Can you work these out from the model? Positions are in its coordinate system, mm. Face numbers are marked on the shaded views. Coordinates: 2 decimals unless noted, no trailing zeros. Order: outer loops, then holes, each group sorted by start corner. A loop starts at its lowest first (then second) coordinate and runs counter-clockwise, first axis right, second up. Notation, with made-up numbers: (9, 36) -> (35, 36) arc R31 cw to (35, 62) -> close; hole circle Ø5 at (-1, -36). An arc over 180 degrees is marked (long way). Answer in a Markdown table with one row per item. Add a question column.
1. We'd pull the mould along X, two halves only. Please class the marked faces 1, 2 and 3: pulls with the +X half, pulls with the -X half, needs draft (parallel to the pull), parting line crosses it, or undercut.
2. Imagine slicing it at A-A on x = 27. Write out the boundary of the cut face in (y, z), plus the area to 3 significant figures.
3. Will these pins go through, and if not, where does the flat tip stop? pin 1 (10 mm diameter, centred on x = 35.5, z = 80.5, fed in from +Y); pin 2 (4 mm diameter, centred on y = 13.5, z = 45, fed in from +X); pin 3 (2 mm diameter, centred on y = 64.5, z = 62.5, fed in from +X).
4. If I drill on line 1 along Y through (x, z) = (20, 29); line 2 along X through (y, z) = (26, 48); line 3 along Y through (x, z) = (42.5, 44), over which ranges is the centre line in solid material (lowest first)? Write a range as [from, to].
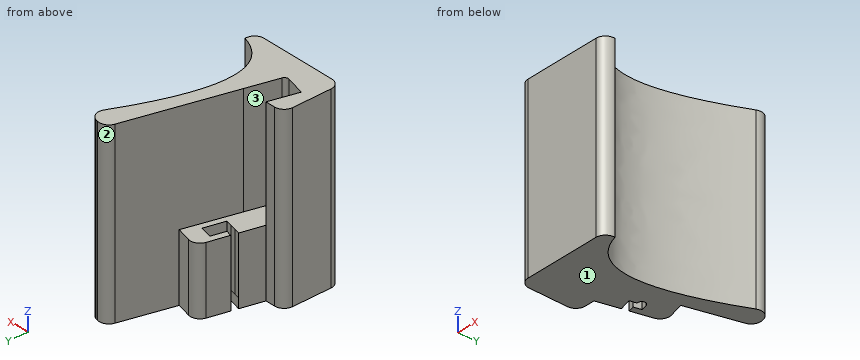
from build123d import *

# Parameters (mm, degrees)
BOSS_EXTRUDE1_DEPTH = 92
BOSS_EXTRUDE2_DEPTH = 5
BOSS_EXTRUDE3_START = 5
BOSS_EXTRUDE3_DEPTH = 30


with BuildPart() as part:
    # Sketch1 → Boss-Extrude1 (new body)
    with BuildSketch(Plane.XY):
        with BuildLine():
            Line((37.386921991, 84.40496063), (22.933554815, 30))
            Line((22.933554815, 30), (18.60433255, 13.818460639))
            ThreePointArc((18.60433255, 13.818460639), (17.672613775, 12.603502297), (16.154645697, 12.403510891))
            Line((16.154645697, 12.403510891), (6.013160809, 15.120913577))
            Line((6.013160809, 15.120913577), (10, 30))
            Line((10, 30), (5, 30))
            ThreePointArc((5, 30), (1.464466094, 28.535533906), (0, 25))
            Line((0, 25), (0, 5))
            ThreePointArc((0, 5), (1.464466094, 1.464466094), (5, 0))
            Line((5, 0), (44.402158914, 0))
            ThreePointArc((44.402158914, 0), (48.110924034, 1.646634335), (49.376897159, 5.501975487))
            add(Edge.make_bspline(
                [(47.769018508, 80.690333507), (37.23731495, 58.823324345), (26.973591169, 24.424922179), (38.309234052, 8.697752331), (49.376897159, 5.501975487)],
                knots=[0.034365073, 0.034365073, 0.034365073, 0.034365073, 0.450207032, 0.866048991, 0.866048991, 0.866048991, 0.866048991], degree=3))
            ThreePointArc((47.769018508, 80.690333507), (47.791234842, 84.982795953), (44.476941442, 87.710649813))
            Line((44.476941442, 87.710649813), (43.43198058, 87.971890028))
            ThreePointArc((43.43198058, 87.971890028), (39.678375933, 87.427416305), (37.386921991, 84.40496063))
        make_face()
    extrude(amount=BOSS_EXTRUDE1_DEPTH)

    # Sketch1_3 → Boss-Extrude2 (add)
    with BuildSketch(Plane.XY):
        with BuildLine():
            Line((22.933554815, 30), (30.160238403, 57.202480315))
            Line((30.160238403, 57.202480315), (22.508418768, 59.201215835))
            ThreePointArc((22.508418768, 59.201215835), (18.694880172, 58.664472736), (16.394052668, 55.576210673))
            Line((16.394052668, 55.576210673), (13.75675976, 45.027039041))
            Line((13.75675976, 45.027039041), (16.890316486, 44.243649859))
            Line((16.890316486, 44.243649859), (17.860458987, 48.12421986))
            Line((17.860458987, 48.12421986), (21.013422112, 47.335979078))
            ThreePointArc((21.013422112, 47.335979078), (22.468635862, 44.910622828), (20.043279612, 43.455409078))
            Line((20.043279612, 43.455409078), (19.194404924, 40.059910327))
            Line((19.194404924, 40.059910327), (12.907885073, 41.63154029))
            Line((12.907885073, 41.63154029), (10, 30))
            Line((10, 30), (6.013160809, 15.120913577))
            Line((6.013160809, 15.120913577), (16.154645697, 12.403510891))
            ThreePointArc((16.154645697, 12.403510891), (17.672613775, 12.603502297), (18.60433255, 13.818460639))
            Line((18.60433255, 13.818460639), (22.933554815, 30))
        make_face()
    extrude(amount=BOSS_EXTRUDE2_DEPTH)

    # Sketch1_4 → Boss-Extrude3 (add)
    with BuildSketch(Plane.XY.offset(BOSS_EXTRUDE3_START)):
        with BuildLine():
            Line((22.933554815, 30), (30.160238403, 57.202480315))
            Line((30.160238403, 57.202480315), (22.508418768, 59.201215835))
            ThreePointArc((22.508418768, 59.201215835), (18.694880172, 58.664472736), (16.394052668, 55.576210673))
            Line((16.394052668, 55.576210673), (14.72690226, 48.907609041))
            Line((14.72690226, 48.907609041), (13.75675976, 45.027039041))
            Line((13.75675976, 45.027039041), (16.890316486, 44.243649859))
            Line((16.890316486, 44.243649859), (17.860458987, 48.12421986))
            Line((17.860458987, 48.12421986), (18.709333674, 51.51971861))
            Line((18.709333674, 51.51971861), (25.015259925, 49.943237047))
            Line((25.015259925, 49.943237047), (22.34736805, 39.271669546))
            Line((22.34736805, 39.271669546), (19.194404924, 40.059910327))
            Line((19.194404924, 40.059910327), (16.041441799, 40.848151108))
            Line((16.041441799, 40.848151108), (12.907885073, 41.63154029))
            Line((12.907885073, 41.63154029), (10, 30))
            Line((10, 30), (6.013160809, 15.120913577))
            Line((6.013160809, 15.120913577), (16.154645697, 12.403510891))
            ThreePointArc((16.154645697, 12.403510891), (17.672613775, 12.603502297), (18.60433255, 13.818460639))
            Line((18.60433255, 13.818460639), (22.933554815, 30))
        make_face()
    extrude(amount=BOSS_EXTRUDE3_DEPTH)


solid = part.part
Answers follow:
| question | item | result |
|---|---|---|
| 1 | face 1 | needs draft |
| 1 | face 2 | parting line crosses it |
| 1 | face 3 | undercut |
| 2 | outline | (0, 0) -> (58.03, 0) -> (58.03, 35) -> (45.31, 35) -> (45.31, 92) -> (0, 92) -> close |
| 2 | area | 4,610 mm² |
| 3 | pin 1 | stops at y = 87.82 |
| 3 | pin 2 | stops at x = 38.76 |
| 3 | pin 3 | stops at x = 41.02 |
| 4 | line 1 | y = [0, 39.86], [51.2, 59.21] |
| 4 | line 2 | x = [0.1, 8.93], [21.86, 32.56] |
| 4 | line 3 | y = [0, 8.51], [69.08, 88.11] |
